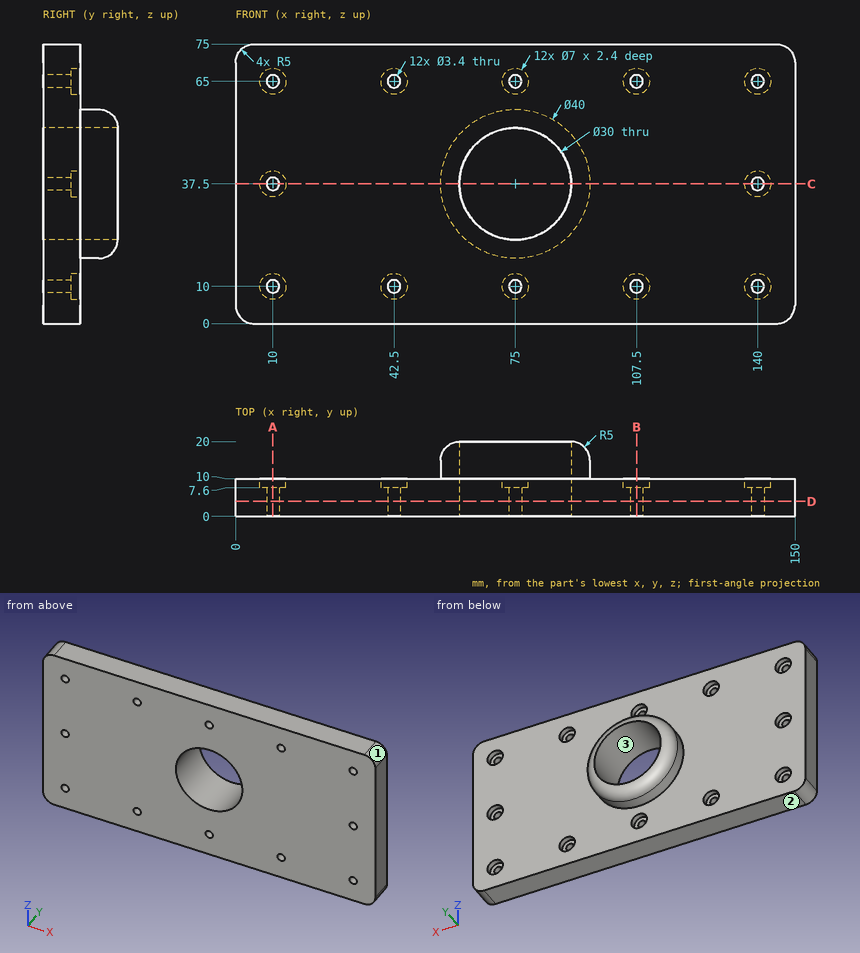
Part print with two shaded views. Sizes in mm from the minimum x, y, z corner. Coordinates: 2 decimals unless noted, no trailing zeros. Order: outer loops, then holes, each group sorted by start corner. A loop starts at its lowest first (then second) coordinate and runs counter-clockwise, first axis right, second up.
(1) Drill centre lines: L1, parallel to X at y = 8.25, z = 65; L2, parallel to Z at x = 10, y = 9.5; L3, parallel to Z at x = 140, y = 2.5. Where is each one in solid material? Low to high.
Solution:
L1: x = 0 to 6.5, 13.5 to 39, 46 to 71.5, 78.5 to 104, 111 to 136.5, 143.5 to 150
L2: z = 0 to 6.5, 13.5 to 34, 41 to 61.5, 68.5 to 75
L3: z = 0 to 8.3, 11.7 to 35.8, 39.2 to 63.3, 66.7 to 75
(2) Mould opens along X. For the marked faces 1, 2 and 3 say: released by +X, released by -X, zero draft, split by the parting line, or undercut.
Solution:
face 1: released by +X
face 2: zero draft
face 3: undercut
(3) Saw through at C-C, the plane z = 37.5. Write the cut outline in (x, y).
Solution:
outline: (0, 0) - (8.3, 0) - (8.3, 7.6) - (6.5, 7.6) - (6.5, 10) - (0, 10) - close; (11.7, 0) - (60, 0) - (60, 20) arc R5 ccw to (55, 15) - (55, 10) - (13.5, 10) - (13.5, 7.6) - (11.7, 7.6) - close; (90, 0) - (138.3, 0) - (138.3, 7.6) - (136.5, 7.6) - (136.5, 10) - (95, 10) - (95, 15) arc R5 ccw to (90, 20) - close; (141.7, 0) - (150, 0) - (150, 10) - (143.5, 10) - (143.5, 7.6) - (141.7, 7.6) - close
(4) Saw through at A-A, the plane x = 10. Write the cut outline in (y, z), and give its area (3 significant figures).
Solution:
outline: (0, 0) - (10, 0) - (10, 6.5) - (7.6, 6.5) - (7.6, 8.3) - (0, 8.3) - close; (0, 11.7) - (7.6, 11.7) - (7.6, 13.5) - (10, 13.5) - (10, 34) - (7.6, 34) - (7.6, 35.8) - (0, 35.8) - close; (0, 39.2) - (7.6, 39.2) - (7.6, 41) - (10, 41) - (10, 61.5) - (7.6, 61.5) - (7.6, 63.3) - (0, 63.3) - close; (0, 66.7) - (7.6, 66.7) - (7.6, 68.5) - (10, 68.5) - (10, 75) - (0, 75) - close
area: 622 mm2
(5) Saw through at D-D, the plane y = 4. Count the separate pieces of the cut face and the enclosed holes in it, and give its area (3 significant figures).
Solution:
separate pieces: 1
enclosed holes: 13
area: 10,400 mm2
(6) Saw through at B-B, the plane x = 107.5. Write the cut outline in (y, z).
Solution:
outline: (0, 0) - (10, 0) - (10, 6.5) - (7.6, 6.5) - (7.6, 8.3) - (0, 8.3) - close; (0, 11.7) - (7.6, 11.7) - (7.6, 13.5) - (10, 13.5) - (10, 61.5) - (7.6, 61.5) - (7.6, 63.3) - (0, 63.3) - close; (0, 66.7) - (7.6, 66.7) - (7.6, 68.5) - (10, 68.5) - (10, 75) - (0, 75) - close
(7) Pin check, flat tips, straight feed: pin 1 Ø11 at (x, z) = (75, 10) entering from +Y; pin 2 Ø1.5 at (y, z) = (15.5, 54.5) entering from -X; pin 3 Ø2 at (x, z) = (76.5, 65.5) entering from +Y. Stop position of each tip, or through.
Solution:
pin 1: stops at y = 10
pin 2: stops at x = 63.38
pin 3: stops at y = 7.6
